CAD build for the part. Positions are in the model's coordinates, mm. Face numbers are marked on the shaded views. A direction names the side the tool comes from. Round coordinates to 2 decimals unless told otherwise and drop trailing zeros. Order: outer loops, then holes, each group sorted by start corner. A loop starts at its lowest first (then second) coordinate and runs counter-clockwise, first axis right, second up. Notation, with made-up numbers: M -19,-14.75 L 7,-14.75 A23 ccw 7,18.25 Z; hole C -2,8.25 d3. An arc over 180 degrees is marked long. Answer as CSV lines item,"result". Start each with the question number.
```python
from build123d import *

# Parameters (mm, degrees)
F1_W     = 101.6
F1_H     = 101.6
F2_DEPTH = 50.8
F3_R     = 12.7
F4_DEPTH = 25.4
F5_R     = 12.7
F6_DEPTH = 17.78


# Not quite as in the source:
# - a variable given as a bare number and used for a length is read in inches; the dataset says mm whatever the document's units were


with BuildPart() as f2:
    # F1 (on Front) → F2 (new body, symmetric)
    with BuildSketch(Plane.XZ):
        Rectangle(F1_W, F1_H)
    extrude(amount=F2_DEPTH, both=True)

    # F3 (on face) → F4 (cut)
    with BuildSketch(Plane.XY.offset(50.8)):
        with Locations((-33.2122892141, 28.3519532531)):
            Circle(F3_R)
    extrude(amount=-F4_DEPTH, mode=Mode.SUBTRACT)

    # F5 (on face) → F6 (join)
    with BuildSketch(Plane(origin=(0, 0, -50.8), x_dir=(1, 0, 0), z_dir=(0, 0, -1))):
        with Locations((-33.2122892141, -28.3519532531)):
            Circle(F5_R)
    extrude(amount=F6_DEPTH)


solid = f2.part
```
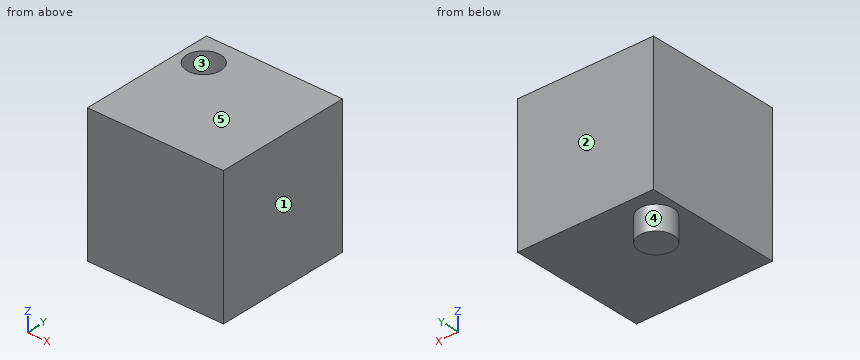
Q1. Probe line 1 along Z through (x, y) = (44.5, -17); line 2 along X through (y, z) = (36, 32). List the from-to ranges inside material, lowest first. Write a range as from..to.
Q2. Band-saw the part on A-A, the plane z = 42.5. Write the cut outline in (x, y), then the cut area to 3 significant figures.
Q3. Band-saw the part on B-B, the plane x = -39. Write the cut outline in (y, z), then the cut area to 3 significant figures.
Q4. Tool access for the marked faces 4 and 5: list every direction of +Z, -Z, +X, -X, +Y, -Y with a clear straight run to the whole face (end or side of a thin tool).
Q5. Drop flat-ended pins along their axis: P1, Ø23, axis at x = -33.21, y = 28.35, coming from the +Z side; P2, Ø12, axis at x = 14.5, y = 40.5, coming from the -Z side. Give the stop position or say it passes through.
Q6. Band-saw the part on C-C, the plane y = -20.5. Write the cut outline in (x, z), then the cut area to 3 significant figures.
Q7. Mould opens along X. For the marked faces 1, 2 and 3 say: +X half, -X half, draft (parallel to the pull), parting line (faces both ways), or undercut.
Answer:
1,line 1,"z = -50.8..50.8"
1,line 2,"x = -50.8..-43.35, -23.07..50.8"
2,outline,"M -50.8,-50.8 L 50.8,-50.8 L 50.8,50.8 L -50.8,50.8 Z; hole C -33.21,28.35 d25.4"
2,area,"9,820 mm^2"
3,outline,"M -50.8,-50.8 L 17.05,-50.8 L 17.05,-68.58 L 39.66,-68.58 L 39.66,-50.8 L 50.8,-50.8 L 50.8,50.8 L 39.66,50.8 L 39.66,25.4 L 17.05,25.4 L 17.05,50.8 L -50.8,50.8 Z"
3,area,"10,200 mm^2"
4,face 4,"-Z"
4,face 5,"+Z, +X, -X, +Y, -Y"
5,P1,"stops at z = 25.4"
5,P2,"stops at z = -50.8"
6,outline,"M -50.8,-50.8 L 50.8,-50.8 L 50.8,50.8 L -50.8,50.8 Z"
6,area,"10,300 mm^2"
7,face 1,"+X half"
7,face 2,"draft"
7,face 3,"undercut"
